Check sheet for the modelled part. Datum: model origin and axes. Units: mm. Round coordinates to 2 decimals unless told otherwise and drop trailing zeros. Write each loop counter-clockwise with the first axis right and the second up, starting at its lowest first coordinate (ties: lowest second). Pieces come first, ordered by that corner, then holes. Notation, with made-up numbers: (4.5, -4) -> (42.5, -4) arc R33 ccw to (42.5, 29) -> close; hole circle Ø11 at (-29.5, 35). An arc over 180 degrees is marked (long way). Write item = value, one per line.
from build123d import *

# Parameters (mm, degrees)
SKETCH_3_R = 1.5


with BuildPart() as part:
    # По траектории1: sweep along a path in Эскиз1
    with BuildLine(Plane(origin=(0, 0, 0), x_dir=(0, 0, -1), z_dir=(1, 0, 0))) as sweep_1_path:
        Line((0, 0), (0, -5))
        ThreePointArc((0, -5), (-0.585786438, -6.414213562), (-2, -7))
        Line((-2, -7), (-6, -7))
        ThreePointArc((-6, -7), (-7.414213562, -7.585786438), (-8, -9))
        Line((-8, -9), (-8, -225))
        ThreePointArc((-8, -225), (-8.585786438, -226.414213562), (-10, -227))
        Line((-10, -227), (-31, -227))
        ThreePointArc((-31, -227), (-32.414213562, -226.414213562), (-33, -225))
        Line((-33, -225), (-33, -192))
    # Эскиз3 → По траектории1 (sweep)
    with BuildSketch(Plane(origin=(0, 0, 0), x_dir=(1, 0, 0), z_dir=(0, 1, 0))):
        Circle(SKETCH_3_R)
    sweep(path=sweep_1_path.line)


solid = part.part
(1) Sectioned sample at C-C on z = 24. Enter the section's corners in (x, y).
Worked answers:
outline = circle Ø3 at (0, -227)
(2) Sectioned sample at A-A on x = 0.9. Enter the section's corners in (y, z).
Worked answers:
outline = (-228.2, 10) arc R3.2 ccw to (-225, 6.8) -> (-9, 6.8) arc R0.8 cw to (-8.2, 6) -> (-8.2, 2) arc R3.2 ccw to (-5, -1.2) -> (0, -1.2) -> (0, 1.2) -> (-5, 1.2) arc R0.8 cw to (-5.8, 2) -> (-5.8, 6) arc R3.2 ccw to (-9, 9.2) -> (-225, 9.2) arc R0.8 cw to (-225.8, 10) -> (-225.8, 31) arc R0.8 cw to (-225, 31.8) -> (-192, 31.8) -> (-192, 34.2) -> (-225, 34.2) arc R3.2 ccw to (-228.2, 31) -> close
(3) Sectioned sample at D-D on y = -55. Enter the section's corners in (x, z).
Worked answers:
outline = circle Ø3 at (0, 8)
(4) Material ranges on L1, parallel to Z at x = 0.3, y = -209; L2, parallel to Z at x = 0.2, y = -47.5; L3, parallel to Z at x = -0.65, y = -204, recorded low to high. Write a range as [from, to].
Worked answers:
L1 = [6.53, 9.47], [31.53, 34.47]
L2 = [6.51, 9.49]
L3 = [6.65, 9.35], [31.65, 34.35]
(5) Go/stop test with flat-tipped pins: P1, Ø12, axis at y = -196.5, z = 16, coming from the +X side; P2, Ø1, axis at x = 0, y = -117, coming from the +Z side. Record where each tip stops, or that it passes through.
Worked answers:
P1 = through
P2 = 9.5
(6) Sectioned sample at B-B on y = -210.5. Enter the section's corners in (x, z), then the cut area to 3 significant figures.
Worked answers:
outline = circle Ø3 at (0, 8); circle Ø3 at (0, 33)
area = 14.1 mm²
